Source: CAD feature listing. Evaluate the final solid. Frame: model axes, mm. Coordinates: 2 decimals unless noted, no trailing zeros. Order: outer loops, then holes, each group sorted by start corner. A loop starts at its lowest first (then second) coordinate and runs counter-clockwise, first axis right, second up. Notation, with made-up numbers: (77.25, 71) -> (89.25, 71) arc R27 ccw to (89.25, 109) -> close; hole circle Ø8 at (-34, 11.25). An arc over 180 degrees is marked (long way). Put each result on its own line as item: value.
from build123d import *

# Parameters (mm, degrees)
F0_W         = 47
F0_H         = 12
F1_DEPTH     = 1.9
F2_W         = 42.6
F2_H         = 7.6
F3_DEPTH     = 2
F4_T4_DEPTH  = 52.9885099991
F4_T9_DEPTH  = 17.9885099991
F4_T14_DEPTH = 52.9885099991
F4_T19_DEPTH = 17.9885099991
F5_R         = 3


# Not quite as in the source:
# - a fillet or chamfer that OpenCascade refuses, or shapes differently, is made with other operations: its cross-section is extruded or revolved along the edge and cut away or added


with BuildPart() as f1:
    # F0 (on Front) → F1 (new body)
    with BuildSketch(Plane.XZ):
        Rectangle(F0_W, F0_H)
    extrude(amount=F1_DEPTH)

    # F2 (on face) → F3 (join)
    with BuildSketch(Plane(origin=(0, 0, 0), x_dir=(-1, 0, 0), z_dir=(0, 1, 0))):
        Rectangle(F2_W, F2_H)
    extrude(amount=F3_DEPTH)

    # F4: chamfer of 0.5 x 2 on 4 edges, made by hand


with BuildPart() as f4_tool2:
    # F4_s3 → F4_t4 (new body)
    with BuildSketch(Plane.YZ.offset(26.4942549995)):
        Polygon((0, -3.8), (2, -3.3), (2, -3.8), align=None)
    extrude(amount=-F4_T4_DEPTH)

    split(bisect_by=Plane.XZ, keep=Keep.BOTTOM)


with BuildPart() as f1_1:
    add(f1.part)

    # F4_t1: cut F4_tool2
    add(f4_tool2.part, mode=Mode.SUBTRACT)


with BuildPart() as f4_tool7:
    # F4_s8 → F4_t9 (new body)
    with BuildSketch(Plane.XY.offset(-8.9942549995)):
        Polygon((-21.3, 0), (-20.8, 2), (-21.3, 2), align=None)
    extrude(amount=F4_T9_DEPTH)

    split(bisect_by=Plane.XZ, keep=Keep.BOTTOM)


with BuildPart() as f1_2:
    add(f1_1.part)

    # F4_t6: cut F4_tool7
    add(f4_tool7.part, mode=Mode.SUBTRACT)


with BuildPart() as f4_tool12:
    # F4_s13 → F4_t14 (new body)
    with BuildSketch(Plane.YZ.offset(-26.4942549995)):
        Polygon((0, 3.8), (2, 3.3), (2, 3.8), align=None)
    extrude(amount=F4_T14_DEPTH)

    split(bisect_by=Plane.XZ, keep=Keep.BOTTOM)


with BuildPart() as f1_3:
    add(f1_2.part)

    # F4_t11: cut F4_tool12
    add(f4_tool12.part, mode=Mode.SUBTRACT)


with BuildPart() as f4_tool17:
    # F4_s18 → F4_t19 (new body)
    with BuildSketch(Plane.XY.offset(8.9942549995)):
        Polygon((21.3, 0), (20.8, 2), (21.3, 2), align=None)
    extrude(amount=-F4_T19_DEPTH)

    split(bisect_by=Plane.XZ, keep=Keep.BOTTOM)


with BuildPart() as f1_4:
    add(f1_3.part)

    # F4_t16: cut F4_tool17
    add(f4_tool17.part, mode=Mode.SUBTRACT)

    # F5
    f5_edges = [f1_4.edges().sort_by_distance(p)[0] for p in [
        (-23.5, -0.95, -6),
        (23.5, -0.95, -6),
        (23.5, -0.95, 6),
        (-23.5, -0.95, 6),
        (-21.05, 1, 3.55),
        (-21.05, 1, -3.55),
        (21.05, 1, 3.55),
        (21.05, 1, -3.55),
    ]]
    fillet(f5_edges, radius=F5_R)


solid = f1_4.part
1. Ray query, line 1 along X through (y, z) = (-1.2, -3.25); line 2 along Y through (x, z) = (21.5, 1.5); line 3 along X through (y, z) = (-1.7, -5.5). Return the intervals inside material, ascending.
Numbers:
line 1: x = -23.49 to 23.49
line 2: y = -1.9 to 0
line 3: x = -22.16 to 22.16
2. Cut plane C-C on z = -4.75. Output: boundary loops of the cut face in (x, y), plus the area to 3 significant figures.
Numbers:
outline: (-22.94, -1.9) -> (22.94, -1.9) -> (22.94, 0) -> (-22.94, 0) -> close
area: 87.2 mm2
3. Cut plane D-D on z = 4.5. Output: boundary loops of the cut face in (x, y).
Numbers:
outline: (-23.1, -1.9) -> (23.1, -1.9) -> (23.1, 0) -> (-23.1, 0) -> close
4. Cut plane A-A on z = 0. Output: boundary loops of the cut face in (x, y), plus the area to 4 significant figures.
Numbers:
outline: (-23.5, -1.9) -> (23.5, -1.9) -> (23.5, 0) -> (21.3, 0) -> (20.8, 2) -> (-20.8, 2) -> (-21.3, 0) -> (-23.5, 0) -> close
area: 173.5 mm2
5. Cut plane B-B on x = -17. Output: boundary loops of the cut face in (y, z), plus the area to 3 significant figures.
Numbers:
outline: (-1.9, -6) -> (0, -6) -> (0, -3.8) -> (2, -3.3) -> (2, 3.3) -> (0, 3.8) -> (0, 6) -> (-1.9, 6) -> close
area: 37.0 mm2
